Check sheet for the modelled part. Datum: model origin and axes. Units: mm. Face numbers are marked on the shaded views. Round coordinates to 2 decimals unless told otherwise and drop trailing zeros. Loops run counter-clockwise (first coordinate to the right, second up) from the corner with the lowest first, then second, coordinate; pieces in that order, holes last. Notation, with made-up numbers: (59.25, 10) - (107.25, 10) arc R21 ccw to (107.25, 28) - close; hole circle Ø1 at (87, 66.25). An arc over 180 degrees is marked (long way). Put each result on its own line as item: value. Start each with the question number.
Item 1: Section check A-A, the plane z = 0. Record the cut outline in (x, y), and give its area (3 significant figures).
Item 2: Gauge pin test, flat ends, axial feed: pin 1 Ø6 at (y, z) = (279, -12) entering from +X; pin 2 Ø5 at (x, y) = (13, 243.5) entering from -Z; pin 3 Ø10 at (x, y) = (6, 284.5) entering from -Z; pin 4 Ø2 at (x, z) = (2.5, 1) entering from -Y. Record the tip position at first contact, or that the pin passes through.
Item 3: Section check C-C, the plane y = 304. Record the cut outline in (x, z).
Item 4: Section check B-B, the plane x = 11. Record the cut outline in (y, z).
Item 5: Draft check along Y on the marked faces 1, 2 and 3. Enter one of: pulls with the +Y half, pulls with the -Y half, needs draft (parallel to the pull), parting line crosses it, or undercut.
Item 6: Material ranges on line 1 along Y through (x, z) = (4, -13); line 2 along Z through (x, y) = (1.5, 24); line 3 along Z through (x, y) = (7, 26.5), recorded low to high.
from build123d import *

# Parameters (mm, degrees)
EXTRUDE_1_DEPTH = 350
EXTRUDE_START   = -2
EXTRUDE_2_DEPTH = 2
EXTRUDE_3_DEPTH = 2


with BuildPart() as part:
    # 草图1 → 凸台-拉伸1 (new body)
    with BuildSketch(Plane(origin=(0, 0, 0), x_dir=(1, 0, 0), z_dir=(0, 1, 0))):
        with BuildLine():
            Line((0, 17), (0, 15))
            ThreePointArc((0, 15), (15, 0), (0, -15))
            Line((0, -15), (0, -17))
            ThreePointArc((0, -17), (17, 0), (0, 17))
        make_face()
    extrude(amount=EXTRUDE_1_DEPTH)

    # 草图2 → 凸台-拉伸2 (add)
    with BuildSketch(Plane(origin=(0, 350, 0), x_dir=(1, 0, 0), z_dir=(0, 1, 0)).offset(EXTRUDE_START)):
        with BuildLine():
            Line((0, 17), (0, 5))
            ThreePointArc((0, 5), (5, 0), (0, -5))
            Line((0, -5), (0, -17))
            ThreePointArc((0, -17), (17, 0), (0, 17))
        make_face()
    extrude(amount=EXTRUDE_2_DEPTH)

    # 草图3 → 凸台-拉伸3 (add)
    with BuildSketch(Plane.XZ):
        with BuildLine():
            Line((0, 17), (0, 5))
            ThreePointArc((0, 5), (5, 0), (0, -5))
            Line((0, -5), (0, -17))
            ThreePointArc((0, -17), (17, 0), (0, 17))
        make_face()
    extrude(amount=-EXTRUDE_3_DEPTH)


solid = part.part
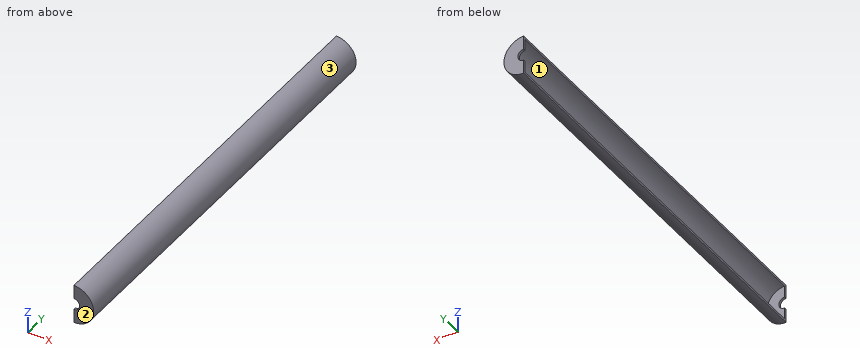
Check result:
1. outline: (5, 0) - (17, 0) - (17, 350) - (5, 350) - (5, 348) - (15, 348) - (15, 2) - (5, 2) - close
1. area: 740 mm²
2. pin 1: x = 14.42
2. pin 2: z = -13.37
2. pin 3: z = -16.97
2. pin 4: through
3. outline: (0, -17) arc R17 ccw to (0, 17) - (0, 15) arc R15 cw to (0, -15) - close
4. outline: (0, -12.96) - (350, -12.96) - (350, 12.96) - (0, 12.96) - close; hole (2, -10.2) - (348, -10.2) - (348, 10.2) - (2, 10.2) - close
5. face 1: undercut
5. face 2: pulls with the -Y half
5. face 3: needs draft
6. line 1: 0 to 2, 348 to 350
6. line 2: -16.93 to -14.92, 14.92 to 16.93
6. line 3: -15.49 to -13.27, 13.27 to 15.49
